```python
from build123d import *

# Parameters (mm, degrees)
SKETCH_1_R          = 27
EXTRUDE_1_DEPTH     = 94
SKETCH_2_R          = 28.4
SKETCH_2_R_2        = 27
EXTRUDE_2_DEPTH     = 20
EXTRUDE_START       = -20
SKETCH_3_R          = 28.4
SKETCH_3_R_2        = 27
EXTRUDE_3_DEPTH     = 20
SKETCH_5_R          = 3
EXTRUDE_4_DEPTH     = 15
SKETCH_9_R          = 4
EXTRUDE_6_DEPTH     = 19.5
SKETCH_10_R         = 12.5
SKETCH_10_R_2       = 4
EXTRUDE_7_DEPTH     = 2
SKETCH_11_R         = 2
CUT_EXTRUDE_2_DEPTH = 2


with BuildPart() as part:
    # 草图1 → 凸台-拉伸1 (new body)
    with BuildSketch(Plane.XY):
        Circle(SKETCH_1_R)
    extrude(amount=-EXTRUDE_1_DEPTH)

    # 草图2 → 凸台-拉伸2 (add)
    with BuildSketch(Plane.XY):
        Circle(SKETCH_2_R)
        Circle(SKETCH_2_R_2, mode=Mode.SUBTRACT)
    extrude(amount=-EXTRUDE_2_DEPTH)

    # 草图3 → 凸台-拉伸3 (add)
    with BuildSketch(Plane(origin=(0, 0, -94), x_dir=(-1, 0, 0), z_dir=(0, 0, -1)).offset(EXTRUDE_START)):
        with Locations(Location((0, 0, 0), (0, 0, 180))):
            Circle(SKETCH_3_R)
        with Locations(Location((0, 0, 0), (0, 0, 180))):
            Circle(SKETCH_3_R_2, mode=Mode.SUBTRACT)
    extrude(amount=EXTRUDE_3_DEPTH)

    # 草图5 → 凸台-拉伸4 (add)
    with BuildSketch(Plane(origin=(0, -20, 0), x_dir=(1, 0, 0), z_dir=(0, 1, 0))):
        with Locations(Location((-7, 84.431486428, 0), (0, 0, 270))):
            Circle(SKETCH_5_R)
        with Locations(Location((7, 84.431486428, 0), (0, 0, 270))):
            Circle(SKETCH_5_R)
    extrude(amount=-EXTRUDE_4_DEPTH)

    # 草图9 → 凸台-拉伸6 (add)
    with BuildSketch(Plane.XY):
        Circle(SKETCH_9_R)
    extrude(amount=EXTRUDE_6_DEPTH)

    # 草图10 → 凸台-拉伸7 (add)
    with BuildSketch(Plane.XY):
        Circle(SKETCH_10_R)
        Circle(SKETCH_10_R_2, mode=Mode.SUBTRACT)
    extrude(amount=EXTRUDE_7_DEPTH)

    # 草图11 → 切除-拉伸2 (cut)
    with BuildSketch(Plane.XY):
        with Locations((19.5, 0)):
            Circle(SKETCH_11_R)
        with Locations((0, 19.5)):
            Circle(SKETCH_11_R)
        with Locations((-19.5, 0)):
            Circle(SKETCH_11_R)
        with Locations((0, -19.5)):
            Circle(SKETCH_11_R)
    extrude(amount=-CUT_EXTRUDE_2_DEPTH, mode=Mode.SUBTRACT)


solid = part.part
```
Geometry check sheet. Reference: the model listing, model coordinates, mm. A direction names the side the tool comes from. Round coordinates to 2 decimals unless told otherwise and drop trailing zeros. Loops run counter-clockwise (first coordinate to the right, second up) from the corner with the lowest first, then second, coordinate; pieces in that order, holes last. Notation, with made-up numbers: (36, -35) - (60, -35) arc R27 ccw to (60, 2) - close; hole circle Ø11 at (68, 61.25). An arc over 180 degrees is marked (long way). Write item = value, one per line. Start each with the question number.
1. Mould release check, pull along Y, two halves, no side actions. Record for faces 1 (the face through (0, -19, -2)), 2 (the face through (-5.85, -26.36, -46.62)), 3 (the face through (25.1, -10.4, -20)), 4 (the face through (7, -35, -84)): released by +Y, released by -Y, zero draft, split by the parting line, or undercut.
2. Set-up check for faces 5 (the face through (-7, -35, -84)), 6 (the face through (10.4, 25.1, -74)), 7 (the face through (0, 20, -2)), 8 (the face through (-9.662, -31.667, -83.047)): record each of +Z, -Z, +X, -X, +Y, -Y from which the full face is reachable in a straight line by a thin tool's end or side.
3. Thickness scan on line 1 (Y direction, x = 0, z = -1.55); line 2 (Z direction, x = -12, y = 25.5); line 3 (Z direction, x = 7, y = 20.5). Record the ranges inside material, lowest first.
4. Section check D-D on x = -19.5. Enter the section's corners in (y, z), then the cut area to 3 significant figures.
5. Section check C-C on z = -42. Enter the section's corners in (x, y), then the cut area to 3 significant figures.
6. Section check A-A on x = 0. Enter the section's corners in (y, z).
7. Depth check by flat-ended pin: pin 1 (3.5 mm diameter, centred on x = 0, y = -19.5, fed in from +Z); pin 2 (4 mm diameter, centred on x = -10, z = -73.5, fed in from -Y); pin 3 (1.5 mm diameter, centred on x = -22, y = 1.5, fed in from +Z). Enter the tip coordinate at first touch or a pass-through.
Working result:
q1.face_1 = undercut
q1.face_2 = split by the parting line
q1.face_3 = zero draft
q1.face_4 = released by -Y
q2.face_5 = +Z, -Z, +X, -X, -Y
q2.face_6 = none
q2.face_7 = +Z
q2.face_8 = -Y
q3.line_1 = -28.4 to -21.5, -17.5 to 17.5, 21.5 to 28.4
q3.line_2 = -94 to -74, -20 to 0
q3.line_3 = -94 to 0
q4.outline = (-20.65, -94) - (20.65, -94) - (20.65, -74) - (18.67, -74) - (18.67, -20) - (20.65, -20) - (20.65, 0) - (2, 0) - (2, -2) - (-2, -2) - (-2, 0) - (-20.65, 0) - (-20.65, -20) - (-18.67, -20) - (-18.67, -74) - (-20.65, -74) - close
q4.area = 3,660 mm^2
q5.outline = circle Ø54 at (0, 0)
q5.area = 2,290 mm^2
q6.outline = (-28.4, -94) - (28.4, -94) - (28.4, -74) - (27, -74) - (27, -20) - (28.4, -20) - (28.4, 0) - (21.5, 0) - (21.5, -2) - (17.5, -2) - (17.5, 0) - (12.5, 0) - (12.5, 2) - (4, 2) - (4, 19.5) - (-4, 19.5) - (-4, 2) - (-12.5, 2) - (-12.5, 0) - (-17.5, 0) - (-17.5, -2) - (-21.5, -2) - (-21.5, 0) - (-28.4, 0) - (-28.4, -20) - (-27, -20) - (-27, -74) - (-28.4, -74) - close
q7.pin_1 = -2
q7.pin_2 = -27.23
q7.pin_3 = 0
